Design review of the part built by this model. Coordinates are the model's own, in mm. A direction names the side the tool comes from. Give positions to 0.01 mm unless a question says otherwise; leave off trailing zeros. Write each loop counter-clockwise with the first axis right and the second up, starting at its lowest first coordinate (ties: lowest second). Pieces come first, ordered by that corner, then holes. Notation, with made-up numbers: (27.25, -0.5) -> (61.25, -0.5) arc R19 ccw to (61.25, 19.5) -> close; hole circle Ø8 at (52.25, -29.5). An arc over 180 degrees is marked (long way). Use CSV: the item, a comma, the result in double quotes.
Solid Edge part; units mm, degrees
sketch "Sketch1" plane through (0, 0, 0) normal (1, 0, 0) x (0, 1, 0)
  line L0 (0, 1.7) -> (2, 1.7)
  line L1 (2, 1.7) -> (2, 12.9)
  arc A0 (2, 12.9) -> (2.3, 13.2) centre (2.3, 12.9) cw
  line L2 (2.3, 13.2) -> (4.7347, 12.7707)
  arc A1 (4.7347, 12.7707) -> (4.9, 12.5737) centre (4.7, 12.5737) cw
  line L3 (4.9, 12.5737) -> (4.9, 11.4)
  line L4 (4.9, 11.4) -> (3.075, 11.4)
  arc A2 (3.075, 11.4) -> (2.7, 11.025) centre (3.075, 11.025) ccw
  line L5 (2.7, 11.025) -> (2.7, 10.6)
  line L6 (2.7, 10.6) -> (3.8293, 10.6)
  line L7 (3.8293, 10.6) -> (3.9, 10.5293)
  line L8 (3.9, 10.5293) -> (3.9, 10.3)
  line L9 (3.9, 10.3) -> (4, 10.3)
  line L10 (4, 10.3) -> (4, 3.2)
  line L11 (4, 3.2) -> (2.75, 1.95)
  line L12 (2.75, 1.95) -> (2.75, 0.6)
  line L13 (2.75, 0.6) -> (2.65, 0.5)
  line L14 (2.65, 0.5) -> (2.75, 0.4)
  line L15 (2.75, 0.4) -> (2.75, 0)
  line L16 (2.75, 0) -> (1.5, 0)
  line L17 (1.5, 0) -> (1.5, -2.1935)
  line L18 (1.5, -2.1935) -> (1.1935, -2.5)
  line L19 (1.1935, -2.5) -> (0, -2.5)
  line L20 (0, -2.5) -> (0, 1.7)
revolve "RevolvedProtrusion1" add sketch "Sketch1" angle 360 about axis through (0, 0, -2.5) along (0, 0, 1)
cosmetic_thread "Thread1"
sketch "Sketch2" plane through (0, 0, -2.5) normal (0, 0, 1) x (1, 0, 0)
  line L0 (-0.75, -0.433) -> (0, -0.866)
  line L1 (0, -0.866) -> (0.75, -0.433)
  line L2 (0.75, -0.433) -> (0.75, 0.433)
  line L3 (0.75, 0.433) -> (0, 0.866)
  line L4 (0, 0.866) -> (-0.75, 0.433)
  line L5 (-0.75, 0.433) -> (-0.75, -0.433)
extrude "ExtrudedCutout_1" cut sketch "Sketch2" along normal blind 4.2
sketch "Sketch3" plane through (0, 0, 13.2) normal (0, 0, 1) x (1, 0, 0)
  line L0 (-10, -10) -> (10, -10)
  line L1 (10, -10) -> (10, 10)
  line L2 (10, 10) -> (-10, 10)
  line L3 (-10, 10) -> (-10, -10)
  line L4 (-3.9, 1) -> (-3.9, -1)
  arc A0 (-3.9, -1) -> (3.9, -1) centre (0, -1) ccw
  line L5 (3.9, -1) -> (3.9, 1)
  arc A1 (3.9, 1) -> (-3.9, 1) centre (0, 1) ccw
extrude "ExtrudedCutout_2" cut sketch "Sketch3" against normal blind 2
properties part number "153314 QSM-M3-4-I"
(1) Take a section at A-A (z = 7.25). Write out the cut boundary in (x, y).
Established:
outline,"circle Ø8 at (0, 0); hole circle Ø4 at (0, 0)"
(2) Take a section at B-B (z = 2.5). Write out the cut boundary in (x, y), then the cut area to 3 significant figures.
Established:
outline,"circle Ø6.6 at (0, 0); hole circle Ø4 at (0, 0)"
area,"21.6 mm2"
(3) Mouldability with a two-part tool opening along Y and no side actions: class faces 1 (the face through (-2.685, -0.596, 1.266)), 2 (the face through (1, 0, 1.7)), 3 (the face through (0.1, 4.9, 12.2)) as +Y half, -Y half, draft (parallel to the pull), parting line (faces both ways), or undercut.
Established:
face 1,"parting line"
face 2,"undercut"
face 3,"+Y half"
(4) Clearance check with flat-ended pins moving along their axes: pin 1 (0.7 mm diameter, centred on y = 0, z = 0, fed in from -X); pin 2 (1.2 mm diameter, centred on y = 0.5, z = 12.5, fed in from +X); pin 3 (1.5 mm diameter, centred on x = 2.5, z = 7.5, fed in from -Y). State where each tip first meets the part, or that it passes through.
Established:
pin 1,"stops at x = -2.75"
pin 2,"stops at x = 3.9"
pin 3,"stops at y = -3.6"
(5) Tool access review of faces 4 (the face through (-0.75, 0, 0)), 5 (the face through (2, 0, 7)), 6 (the face through (1, -3, 10.6)), 7 (the face through (0.07, -1.5, -1.11)): name each direction out of +Z, -Z, +X, -X, +Y, -Y from which nothing blocks a thin tool from reaching the whole face with its end or side.
Established:
face 4,"+Z, -Z"
face 5,"+Z"
face 6,"none"
face 7,"-Z"
(6) For line 1 along X through (y, z) = (0, 4.75); line 2 along Y through (x, z) = (0, 11.5), list the stretches that pass through material, from the lowest coordinate up. Write a range as [from, to].
Established:
line 1,"x = [-4, -2], [2, 4]"
line 2,"y = [-4.9, -2], [2, 4.9]"
